The figure shows three views and two pictorial views of one solid part (mm, origin at its lowest corner). Answer the questions. A direction names the side the tool comes from. Round coordinates to 2 decimals unless told otherwise and drop trailing zeros. Order: outer loops, then holes, each group sorted by start corner. A loop starts at its lowest first (then second) coordinate and runs counter-clockwise, first axis right, second up. Notation, with made-up numbers: (53.5, 59.25) -> (59.5, 59.25) arc R24 ccw to (59.5, 96.25) -> close; hole circle Ø3 at (-16.5, 10). An arc over 180 degrees is marked (long way). Return JSON: item names as keys, results as strings. Group by question number.
(1) The part is cut by section D-D (x = 15.5). Determine the outline of the cut face in (y, z) (1 decimal).
(2) Which of the six approach directions +Z, -Z, +X, -X, +Y, -Y give full straight-line access (tool end or side, diameter ignored) to the marked faces 1 and 2?
(3) The part is cut by section B-B (y = 14). Determine the outline of the cut face in (x, z).
(4) Consider line 1 (Y direction, x = 20.5, z = 1.05); line 2 (Y direction, x = 22.5, z = 0.5); line 3 (X direction, y = 7.5, z = 1.85). Determine where each line is inside the solid, lowest interval first. Write a range as [from, to].
(5) The part is cut by section A-A (x = 22). Determine the outline of the cut face in (y, z).
(6) Each of these flat-tipped pins is pushed along its axis until it touches: pin 1 (1.5 mm diameter, centred on x = 15, z = 1.5, fed in from -Y); pin 2 (1 mm diameter, centred on y = 5, z = 1, fed in from +X). Where does it stop, or does it pass through?
(7) Determine the mould class of the marked faces 3, 4, 5 and 6 for opening direction Y: +Y half, -Y half, draft (parallel to the pull), parting line (faces both ways), or undercut.
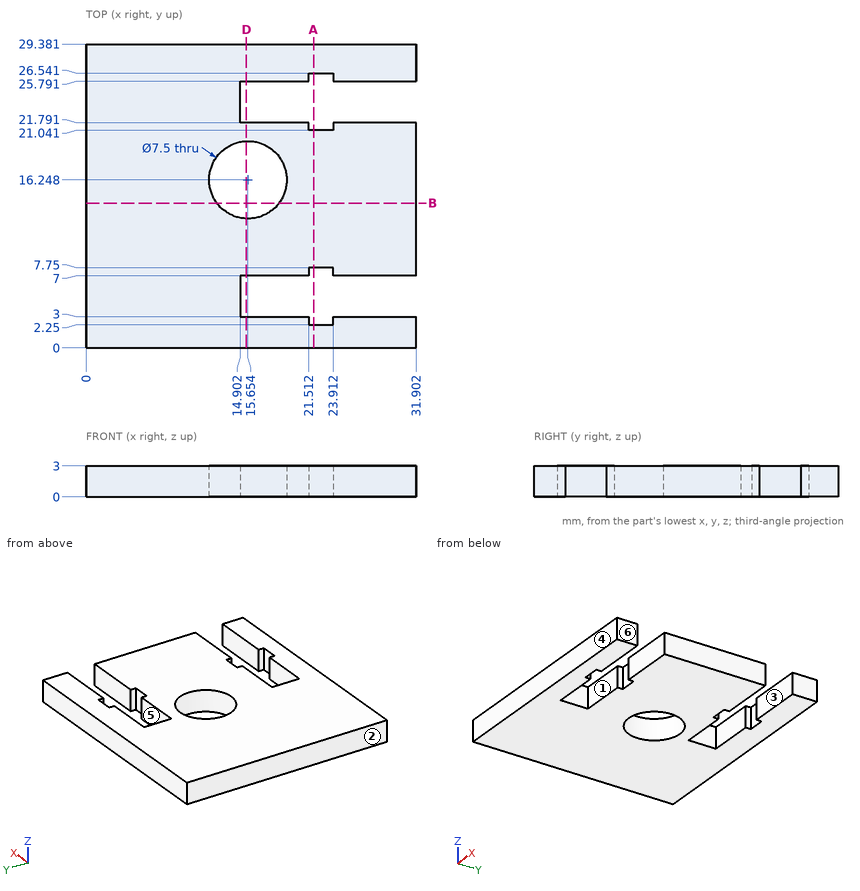
Answer below:
{
 "1": {"outline": "(0, 0) -> (3, 0) -> (3, 3) -> (0, 3) -> close; (7, 0) -> (12.5, 0) -> (12.5, 3) -> (7, 3) -> close; (20, 0) -> (21.8, 0) -> (21.8, 3) -> (20, 3) -> close; (25.8, 0) -> (29.4, 0) -> (29.4, 3) -> (25.8, 3) -> close"},
 "2": {"face 1": "+Z, -Z, +X", "face 2": "+Z, -Z, -X, +Y, -Y"},
 "3": {"outline": "(0, 0) -> (12.65, 0) -> (12.65, 3) -> (0, 3) -> close; (18.66, 0) -> (31.9, 0) -> (31.9, 3) -> (18.66, 3) -> close"},
 "4": {"line 1": "y = [0, 3], [7, 21.79], [25.79, 29.38]", "line 2": "y = [0, 2.25], [7.75, 21.04], [26.54, 29.38]", "line 3": "x = [0, 21.51], [23.91, 31.9]"},
 "5": {"outline": "(0, 0) -> (2.25, 0) -> (2.25, 3) -> (0, 3) -> close; (7.75, 0) -> (21.04, 0) -> (21.04, 3) -> (7.75, 3) -> close; (26.54, 0) -> (29.38, 0) -> (29.38, 3) -> (26.54, 3) -> close"},
 "6": {"pin 1": "stops at y = 0", "pin 2": "stops at x = 14.9"},
 "7": {"face 3": "undercut", "face 4": "-Y half", "face 5": "undercut", "face 6": "draft"}
}
